Autodesk Inventor part; units mm, degrees
ref_plane "YZ Plane" through (0, 0, 0) normal (1, 0, 0) x (0, 1, 0)
ref_plane "XZ Plane" through (0, 0, 0) normal (0, 1, 0) x (-1, 0, 0)
ref_plane "XY Plane" through (0, 0, 0) normal (0, 0, 1) x (1, 0, 0)
sketch "Sketch1" plane through (0, 0, 0) normal (0, 0, 1) x (1, 0, 0)
  line L0 (0, 0) -> (600, 0)
  line L1 (600, 0) -> (600, -93)
  line L2 (600, -93) -> (0, -93)
  line L3 (0, -93) -> (0, 0)
  line L4 (100, -93) -> (500, -93)
  line L5 (500, -93) -> (500, -223)
  line L6 (500, -223) -> (100, -223)
  line L7 (100, -223) -> (100, -93)
  point P0 (300, -93)
  point P1 (300, -223)
  dimension "d0" = 600
  dimension "d1" = 93
  dimension "d2" = 400
  dimension "d6" = 223
extrude "Extrusion1" add sketch "Sketch1" along normal blind 10
properties part number "Front Cover" material "ABS Plastic"
Verification items for the finished model (mm, model axes). A direction names the side the tool comes from. Coordinates: 2 decimals unless noted, no trailing zeros. Order: outer loops, then holes, each group sorted by start corner. A loop starts at its lowest first (then second) coordinate and runs counter-clockwise, first axis right, second up. Notation, with made-up numbers: (-31, 61) -> (6, 61) arc R18 ccw to (6, 93) -> close; hole circle Ø2 at (67.25, 39.5). An arc over 180 degrees is marked (long way). Put each result on its own line as item: value. Start each with the question number.
1. Cross-section at C-C, the plane x = 58.5. Record the boundary of the cut face in (y, z), then the cut area to 3 significant figures.
2. Access from +Z, -Z, +X, -X, +Y, -Y to the whole of each face (thin tool, end or side, straight path). Record for faces 1 (the flat face through (51, -93, 5)), 2 (the flat face through (551, -93, 5)), 3 (the flat face through (0, -47, 5)).
3. Material ranges on L1, parallel to Y at x = 569, z = 0.5; L2, parallel to X at y = -136, z = 9.5, recorded low to high. Write a range as [from, to].
4. Go/stop test with flat-tipped pins: pin 1 Ø5 at (y, z) = (-139.5, 4.5) entering from -X; pin 2 Ø3 at (y, z) = (-184, 6) entering from +X; pin 3 Ø3 at (x, z) = (558, 6.5) entering from -Y. Record where each tip stops, or that it passes through.
5. Cross-section at B-B, the plane y = -130. Record the boundary of the cut face in (x, z).
6. Cross-section at A-A, the plane z = 3.5. Record the boundary of the cut face in (x, y), then the cut area to 3 significant figures.
Computed:
1. outline: (-93, 0) -> (0, 0) -> (0, 10) -> (-93, 10) -> close
1. area: 930 mm2
2. face 1: +Z, -Z, -X, -Y
2. face 2: +Z, -Z, +X, -Y
2. face 3: +Z, -Z, -X, +Y, -Y
3. L1: [-93, 0]
3. L2: [100, 500]
4. pin 1: x = 100
4. pin 2: x = 500
4. pin 3: y = -93
5. outline: (100, 0) -> (500, 0) -> (500, 10) -> (100, 10) -> close
6. outline: (0, -93) -> (100, -93) -> (100, -223) -> (500, -223) -> (500, -93) -> (600, -93) -> (600, 0) -> (0, 0) -> close
6. area: 108,000 mm2
